Work out the finished part from the listing and answer in its coordinate system (mm). A direction names the side the tool comes from. Give positions to 0.01 mm unless a question says otherwise; leave off trailing zeros. Write each loop counter-clockwise with the first axis right and the second up, starting at its lowest first coordinate (ties: lowest second). Pieces come first, ordered by that corner, then holes.
1) A tool of negligible diameter and unlimited length cuts with its end or side. For faces 5 (the face through (195.5, -15.3, 1.2)), 6 (the face through (-286.2, -12.65, 8.06)), 7 (the face through (-235.5, -15.3, -1.2)), 8 (the face through (333.979, -4.506, 14.307)), from which of +Z, -Z, +X, -X, +Y, -Y can it reach the whole face along a straight path? Write none if from no direction.
2) Find section C-C (x = -267.5). Determine the outline of the cut face in (y, z), plus the area to 3 significant figures.
3) Given pin 1 Ø3 at (x, z) = (216.5, -5.5) entering from -Y; pin 2 Ø5 at (x, y) = (-244.5, -12.5) entering from +Z; pin 3 Ø5 at (x, y) = (12.5, 8.5) entering from +Z, each flat-ended and moving along its own axis, determine where each tip first touches the part or whether it passes through.
4) Find section A-A (z = 0). Determine the outline of the cut face in (x, y).
5) Find section B-B (x = -28). Determine the outline of the cut face in (y, z).
6) Determine the mould class of faces 1 (the face through (-23.02, -17.5, 0.25)), 2 (the face through (-235.5, 15.2, -0.1)), 3 (the face through (335.5, 0, 0)), 4 (the face through (331.71, -13.98, -3)) for opening direction X: pulls with the +X half, pulls with the -X half, needs draft (parallel to the pull), parting line crosses it, or undercut.
7) Straight lines are drawn through the part: probe 1 along X at (y, z) = (-13.5, -5); probe 2 along Z at (x, y) = (-65, -4); probe 3 along X at (y, z) = (-9.5, 12). For each, find the intervals that lie inside material, in ascending order.
```python
from build123d import *

# Parameters (mm, degrees)
CUT_EXTRUDE1_DEPTH = 431
SKETCH3_W          = 1.6
SKETCH3_H          = 0.7
CUT_EXTRUDE2_DEPTH = 5


with BuildPart() as part:
    # Sketch1 → Revolve1 (revolve)
    with BuildSketch(Plane.XY, mode=Mode.PRIVATE) as revolve1_sk:
        Polygon((-335.5, 0), (335.5, 0), (335.5, 15), (195.5, 15), (195.5, 17.5), (-235.5, 17.5), (-235.5, 15), (-335.5, 15), align=None)
    revolve(revolve1_sk.sketch.rotate(Axis((-335.5, 0, 0), (1, 0, 0)), 90), axis=Axis((-335.5, 0, 0), (1, 0, 0)))

    # Sketch2 → Cut-Extrude1 (cut)
    with BuildSketch(Plane.ZY.offset(235.5)):
        with BuildLine():
            Line((-14.936600675, 9.118550338), (-15.062665819, -8.908765258))
            ThreePointArc((-15.062665819, -8.908765258), (-17.499572122, 0.12237463), (-14.936600675, 9.118550338))
        make_face()
        with BuildLine():
            Line((14.936600675, 9.118550338), (15.062665819, -8.908765258))
            ThreePointArc((15.062665819, -8.908765258), (17.499572122, 0.12237463), (14.936600675, 9.118550338))
        make_face()
    extrude(amount=-CUT_EXTRUDE1_DEPTH, mode=Mode.SUBTRACT)

    # Sketch3 → Cut-Revolve1 (revolve, cut)
    with BuildSketch(Plane(origin=(0, 0, 0), x_dir=(1, 0, 0), z_dir=(0, 1, 0)), mode=Mode.PRIVATE) as cut_revolve1_sk:
        with Locations((331.7, 14.65)):
            Rectangle(SKETCH3_W, SKETCH3_H)
    revolve(cut_revolve1_sk.sketch.rotate(Axis((335.5, 0, 0), (-1, 0, 0)), 180.400663256), axis=Axis((335.5, 0, 0), (-1, 0, 0)), mode=Mode.SUBTRACT)

    # Sketch6 → Cut-Extrude2 (cut)
    with BuildSketch(Plane(origin=(0, 1.378544902, -14.936519473), x_dir=(0, -0.9957679648377556, -0.09190299343804982), z_dir=(0, -0.09190299343804982, 0.9957679648377556))):
        with BuildLine():
            Line((5, 322.5), (5, 292.5))
            ThreePointArc((5, 292.5), (0, 287.5), (-5, 292.5))
            Line((-5, 292.5), (-5, 322.5))
            ThreePointArc((-5, 322.5), (0, 327.5), (5, 322.5))
        make_face()
    extrude(amount=CUT_EXTRUDE2_DEPTH, mode=Mode.SUBTRACT)


solid = part.part
```
Results:
1. face 5: +X, -Y
1. face 6: -X
1. face 7: -X, -Y
1. face 8: +X
2. outline: circle Ø30 at (0, 0)
2. area: 707 mm2
3. pin 1: stops at y = -14.46
3. pin 2: stops at z = 11.18
3. pin 3: stops at z = 14.96
4. outline: (-335.5, -15) - (-235.5, -15) - (-235.5, -17.5) - (195.5, -17.5) - (195.5, -15) - (330.9, -15) - (330.9, -14.3) - (332.5, -14.3) - (332.5, -15) - (335.5, -15) - (335.5, 15) - (332.5, 15) - (332.5, 14.3) - (330.9, 14.3) - (330.9, 15) - (195.5, 15) - (195.5, 17.5) - (-235.5, 17.5) - (-235.5, 15) - (-335.5, 15) - close
5. outline: (-8.91, -15.06) - (9.12, -14.94) arc R17.5 ccw to (9.12, 14.94) - (-8.91, 15.06) arc R17.5 ccw to start
6. face 1: needs draft
6. face 2: pulls with the -X half
6. face 3: pulls with the +X half
6. face 4: undercut
7. probe 1: x = -335.5 to 330.9, 332.5 to 335.5
7. probe 2: z = -15.03 to 15.03
7. probe 3: x = -235.5 to 195.5
